from build123d import *

# Parameters (mm, degrees)
SKETCH1_W           = 337
SKETCH1_H           = 10
BOSS_EXTRUDE1_DEPTH = 5
SKETCH2_W           = 337
SKETCH2_H           = 2.5
BOSS_EXTRUDE2_DEPTH = 5
SKETCH3_W           = 337
SKETCH3_H           = 2.5
BOSS_EXTRUDE3_DEPTH = 15
SKETCH4_R           = 2.5
BOSS_EXTRUDE4_DEPTH = 20


with BuildPart() as part:
    # Sketch1 → Boss-Extrude1 (new body)
    with BuildSketch(Plane(origin=(0, 0, 0), x_dir=(1, 0, 0), z_dir=(0, 1, 0))):
        Rectangle(SKETCH1_W, SKETCH1_H)
    extrude(amount=BOSS_EXTRUDE1_DEPTH)

    # Sketch2 → Boss-Extrude2 (add)
    with BuildSketch(Plane(origin=(0, 5, 0), x_dir=(1, 0, 0), z_dir=(0, 1, 0))):
        with Locations((0, -3.75)):
            Rectangle(SKETCH2_W, SKETCH2_H)
    extrude(amount=BOSS_EXTRUDE2_DEPTH)

    # Sketch3 → Boss-Extrude3 (add)
    with BuildSketch(Plane(origin=(0, 5, 0), x_dir=(1, 0, 0), z_dir=(0, 1, 0))):
        with Locations((0, 3.75)):
            Rectangle(SKETCH3_W, SKETCH3_H)
    extrude(amount=BOSS_EXTRUDE3_DEPTH)

    # Sketch4 → Boss-Extrude4 (add)
    with BuildSketch(Plane.XZ):
        with Locations((-158.5, 0)):
            Circle(SKETCH4_R)
        with Locations((158.5, 0)):
            Circle(SKETCH4_R)
    extrude(amount=BOSS_EXTRUDE4_DEPTH)


solid = part.part
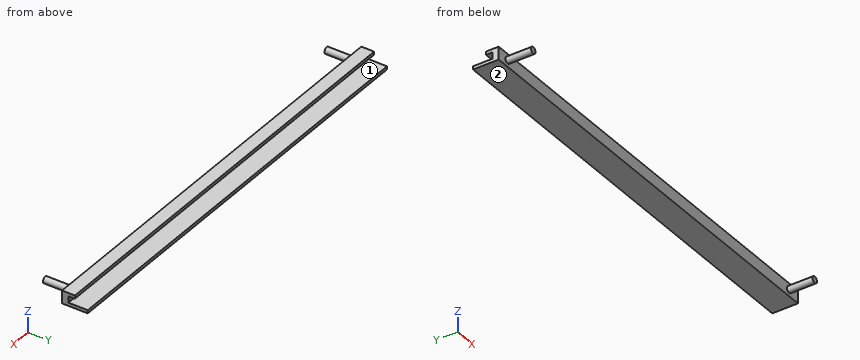
Verification items for the finished model (mm, model axes). Face numbers are marked on the shaded views. Give positions to 0.01 mm unless a question says otherwise; leave off trailing zeros. Order: outer loops, then holes, each group sorted by start corner. A loop starts at its lowest first (then second) coordinate and runs counter-clockwise, first axis right, second up. Notation, with made-up numbers: M 74.25,17.25 L 81.25,17.25 A22 cw 81.25,26.25 Z; hole C -16,-1 d3. An arc over 180 degrees is marked long. Answer as a JSON object with one key per item and string values. Group by question number.
1) Mould release check, pull along Z, two halves, no side actions. Record for the marked faces 1 and 2: released by +Z, released by -Z, zero draft, split by the parting line, or undercut.
2) Depth check by flat-ended pin: pin 1 Ø2 at (x, z) = (-20.5, 3.5) entering from +Y; pin 2 Ø5 at (y, z) = (-10, -1) entering from -X; pin 3 Ø4 at (y, z) = (-3, -2) entering from +X. Enter the tip coordinate at first touch or a pass-through.
3) Cross-section at B-B (z = 0). Enter the section's corners in (x, y), then the cut area to 4 significant figures.
4) Cross-section at A-A (x = 145). Enter the section's corners in (y, z), then the cut area to 3 significant figures.
5) Scan lines: line 1 along X through (y, z) = (-0.5, 0.5); line 2 along Y through (x, z) = (72, 3.5); line 3 along Y through (x, z) = (89, -1.5). Record each from-to range of solid material in increasing order. Write a range as [from, to].
6) Cross-section at C-C (y = 14). Enter the section's corners in (x, z), then the cut area to 4 significant figures.
Result sheet:
{
 "1": {"face 1": "undercut", "face 2": "released by -Z"},
 "2": {"pin 1": "stops at y = 10", "pin 2": "stops at x = -161", "pin 3": "stops at x = 161"},
 "3": {"outline": "M -168.5,0 L -161,0 L -161,-20 L -156,-20 L -156,0 L 156,0 L 156,-20 L 161,-20 L 161,0 L 168.5,0 L 168.5,5 L -168.5,5 Z", "area": "1,885 mm2"},
 "4": {"outline": "M 0,-5 L 20,-5 L 20,-2.5 L 5,-2.5 L 5,2.5 L 10,2.5 L 10,5 L 0,5 Z", "area": "100 mm2"},
 "5": {"line 1": "x = [-160.95, -156.05], [156.05, 160.95]", "line 2": "y = [0, 10]", "line 3": "y = [0, 5]"},
 "6": {"outline": "M -168.5,-5 L 168.5,-5 L 168.5,-2.5 L -168.5,-2.5 Z", "area": "842.5 mm2"}
}
